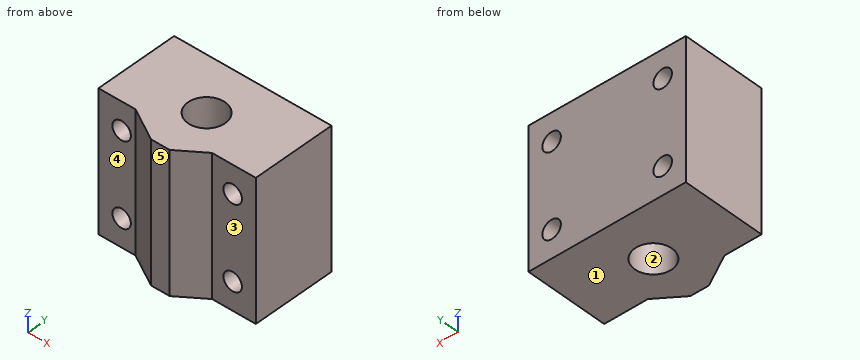
```python
from build123d import *

# Parameters (mm, degrees)
SKETCH2_R           = 4
BOSS_EXTRUDE1_DEPTH = 30
SKETCH4_R           = 2
CUT_EXTRUDE1_DEPTH  = 19


with BuildPart() as part:
    # Sketch2 → Boss-Extrude1 (new body)
    with BuildSketch(Plane.XY):
        Polygon((0, 0), (34, 0), (34, -18), (27.548015077, -18), (24.548015077, -18), (19, -22), (17, -22), (15, -22), (8, -18), (5, -18), (0, -18), align=None)
        with Locations((17, -11)):
            Circle(SKETCH2_R, mode=Mode.SUBTRACT)
    extrude(amount=BOSS_EXTRUDE1_DEPTH)

    # Sketch4 → Cut-Extrude1 (cut, through all)
    with BuildSketch(Plane.XZ.offset(18)):
        with Locations((5, 6)):
            Circle(SKETCH4_R)
        with Locations((29, 6)):
            Circle(SKETCH4_R)
        with Locations((5, 24)):
            Circle(SKETCH4_R)
        with Locations((29, 24)):
            Circle(SKETCH4_R)
    extrude(amount=-CUT_EXTRUDE1_DEPTH, mode=Mode.SUBTRACT)


solid = part.part
```
The listing builds one solid part. Answer for the finished solid, in the listing's coordinates (mm). Face numbers are marked on the shaded views. A direction names the side the tool comes from. Round coordinates to 2 decimals unless told otherwise and drop trailing zeros. Loops run counter-clockwise (first coordinate to the right, second up) from the corner with the lowest first, then second, coordinate; pieces in that order, holes last. Notation, with made-up numbers: (-21, -0.75) - (-2, -0.75) arc R34 cw to (-2, 34.25) - close; hole circle Ø7 at (79, 31). An arc over 180 degrees is marked (long way). Use one line per item in the form item = value. Start each with the question number.
1. The part is cut by section A-A on z = 6. Determine the outline of the cut face in (x, y), then the cut area to 3 significant figures.
2. Consider line 1 (Z direction, x = 29, y = -3.5); line 2 (X direction, y = -3.5, z = 23.5); line 3 (Y direction, x = 17, z = 24). Determine where each line is inside the solid, lowest interval first. Write a range as [from, to].
3. A tool of negligible diameter and unlimited length cuts with its end or side. For the marked faces 4 and 5, from which of +Z, -Z, +X, -X, +Y, -Y can it reach the whole face along a straight path? Write none if from no direction.
4. The part is cut by section B-B on x = 17. Determine the outline of the cut face in (y, z).
5. The part is cut by section D-D on x = 5. Determine the outline of the cut face in (y, z).
6. For a pull along Y with two mould halves and no side action, classify the marked faces 1, 2 and 3 as pulls with the +Y half, pulls with the -Y half, needs draft (parallel to the pull), parting line crosses it, or undercut.
7. Given pin 1 Ø3.5 at (x, z) = (5, 6) entering from +Y; pin 2 Ø4.5 at (x, z) = (29.5, 16) entering from -Y, each flat-ended and moving along its own axis, determine where each tip first touches the part or whether it passes through.
8. The part is cut by section C-C on z = 21.25. Determine the outline of the cut face in (x, y).
Geometry check:
q1.outline = (0, -18) - (3, -18) - (3, 0) - (0, 0) - close; (7, -18) - (8, -18) - (15, -22) - (19, -22) - (24.55, -18) - (27, -18) - (27, 0) - (7, 0) - close; (31, -18) - (34, -18) - (34, 0) - (31, 0) - close; hole circle Ø8 at (17, -11)
q1.area = 459 mm^2
q2.line_1 = [0, 4], [8, 22], [26, 30]
q2.line_2 = [0, 3.06], [6.94, 27.06], [30.94, 34]
q2.line_3 = [-22, -15], [-7, 0]
q3.face_4 = +Z, -Z, -X, -Y
q3.face_5 = +Z, -Z, +X, -X, -Y
q4.outline = (-22, 0) - (-15, 0) - (-15, 30) - (-22, 30) - close; (-7, 0) - (0, 0) - (0, 30) - (-7, 30) - close
q5.outline = (-18, 0) - (0, 0) - (0, 4) - (-18, 4) - close; (-18, 8) - (0, 8) - (0, 22) - (-18, 22) - close; (-18, 26) - (0, 26) - (0, 30) - (-18, 30) - close
q6.face_1 = needs draft
q6.face_2 = undercut
q6.face_3 = pulls with the -Y half
q7.pin_1 = through
q7.pin_2 = -18
q8.outline = (0, -18) - (8, -18) - (15, -22) - (19, -22) - (24.55, -18) - (34, -18) - (34, 0) - (0, 0) - close; hole circle Ø8 at (17, -11)
